For this review, use the dimensioned drawing (mm, ordinates from the lowest corner) and the shaded views. Give positions to 0.01 mm unless a question says otherwise; leave off trailing zeros. Order: outer loops, then holes, each group sorted by start corner. A loop starts at its lowest first (then second) coordinate and runs counter-clockwise, first axis right, second up. Notation, with made-up numbers: (59, 65.25) - (76, 65.25) arc R14 ccw to (76, 83.25) - close; hole circle Ø2 at (-14.75, -23.75). An arc over 180 degrees is marked (long way). Use a Markdown table: item, result. Add a question column.
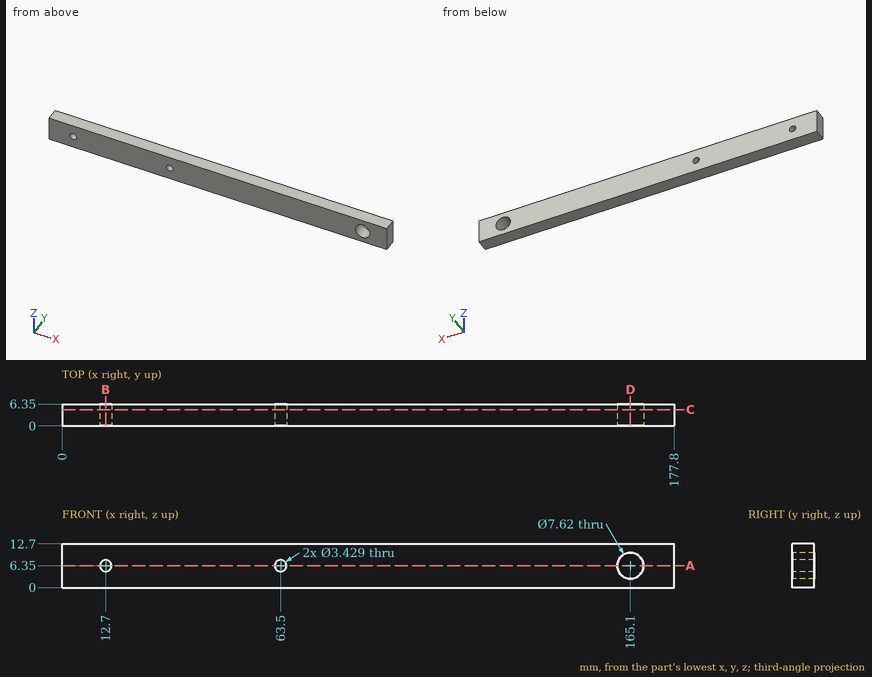
Q1. We need section B-B (x = 12.7). Write out the cut boundary in (y, z).
Q2. We need section C-C (y = 4.75). Write out the cut boundary in (x, z), plus the area to 3 significant figures.
Q3. Wall thickness on probe 1 along Z at (x, y) = (12.7, 4.5); probe 2 along Z at (x, y) = (165.1, 5); probe 3 along X at (y, z) = (0.75, 8.75): over which ranges is each line inside the solid? List them lowest first.
Q4. We need section D-D (x = 165.1). Write out the cut boundary in (y, z).
Q5. Clearance check with a flat-ended pin moving along its axis: P1, Ø2, axis at x = 12.7, z = 6.35, coming from the +Y side. State where the tip first meets the part, or that it passes through.
Q6. We need section A-A (z = 6.35). Write out the cut boundary in (x, y), plus the area to 3 significant figures.
Here are the results:
| question | item | result |
|---|---|---|
| 1 | outline | (0, 0) - (6.35, 0) - (6.35, 4.64) - (0, 4.64) - close; (0, 8.06) - (6.35, 8.06) - (6.35, 12.7) - (0, 12.7) - close |
| 2 | outline | (0, 0) - (177.8, 0) - (177.8, 12.7) - (0, 12.7) - close; hole circle Ø3.43 at (12.7, 6.35); hole circle Ø3.43 at (63.5, 6.35); hole circle Ø7.62 at (165.1, 6.35) |
| 2 | area | 2,190 mm2 |
| 3 | probe 1 | 0 to 4.64, 8.06 to 12.7 |
| 3 | probe 2 | 0 to 2.54, 10.16 to 12.7 |
| 3 | probe 3 | 0 to 162.14, 168.06 to 177.8 |
| 4 | outline | (0, 0) - (6.35, 0) - (6.35, 2.54) - (0, 2.54) - close; (0, 10.16) - (6.35, 10.16) - (6.35, 12.7) - (0, 12.7) - close |
| 5 | P1 | through |
| 6 | outline | (0, 0) - (10.99, 0) - (10.99, 6.35) - (0, 6.35) - close; (14.41, 0) - (61.79, 0) - (61.79, 6.35) - (14.41, 6.35) - close; (65.21, 0) - (161.29, 0) - (161.29, 6.35) - (65.21, 6.35) - close; (168.91, 0) - (177.8, 0) - (177.8, 6.35) - (168.91, 6.35) - close |
| 6 | area | 1,040 mm2 |
